```python
from build123d import *

# Parameters (mm, degrees)
F2_R     = 4.2169292551
F3_DEPTH = 41.402
F4_R     = 3.4205639175
F5_DEPTH = 25.4
F6_W     = 9.9848257378
F6_H     = 8.4082745016
F7_DEPTH = 41.402
F8_W     = 6.5733380616
F8_H     = 5.3974576294
F9_DEPTH = 25.4


# Not quite as in the source:
# - the program builds the solid bodies; features that only make, move or delete a surface that nothing else refers to are left out


with BuildPart() as f3:
    # F2 (on Right) → F3 (new body)
    with BuildSketch(Plane.YZ):
        with Locations((0, -23.187154904)):
            Circle(F2_R)
    extrude(amount=F3_DEPTH)

    # F4 (on face) → F5 (cut)
    with BuildSketch(Plane.YZ.offset(41.402)):
        with Locations((0, -23.187154904)):
            Circle(F4_R)
    extrude(amount=-F5_DEPTH, mode=Mode.SUBTRACT)

    # F6 (on Right) → F7 (join)
    with BuildSketch(Plane.YZ):
        with Locations((0, -23.9110346884)):
            Rectangle(F6_W, F6_H)
    extrude(amount=-F7_DEPTH)

    # F8 (on face) → F9 (cut)
    with BuildSketch(Plane(origin=(-41.402, 0, 0), x_dir=(0, -1, 0), z_dir=(-1, 0, 0))):
        with Locations((0, -23.9110346884)):
            Rectangle(F8_W, F8_H)
    extrude(amount=-F9_DEPTH, mode=Mode.SUBTRACT)


solid = f3.part
```
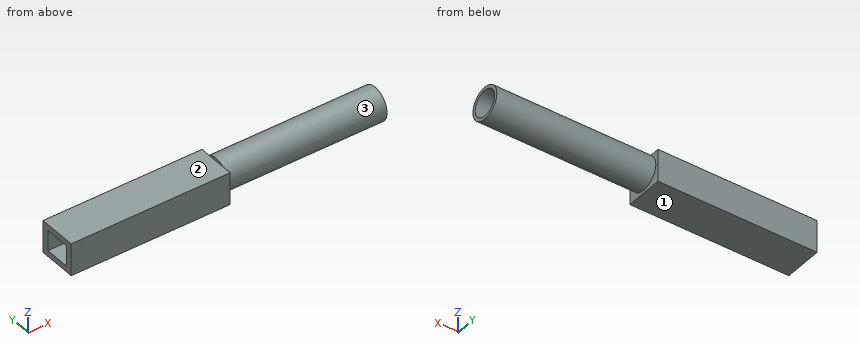
The listing builds one solid part. Answer for the finished solid, in the listing's coordinates (mm). Face numbers are marked on the shaded views. A direction names the side the tool comes from. Round coordinates to 2 decimals unless told otherwise and drop trailing zeros. Write each loop counter-clockwise with the first axis right and the second up, starting at its lowest first coordinate (ties: lowest second). Pieces come first, ordered by that corner, then holes. Notation, with made-up numbers: (70.5, -15) -> (126.5, -15) arc R13 cw to (126.5, -10) -> close; hole circle Ø6 at (53.5, 2.25). An arc over 180 degrees is marked (long way). Answer as a JSON object with one key per item and string values. Group by question number.
Q1. Section B-B (y = 0) is taken. Write down the section's boundary in (x, z).
Q2. Section C-C (z = -20.5) is taken. Write down the section's boundary in (x, y), plus the area to 3 significant figures.
Q3. Which of the six approach directions +Z, -Z, +X, -X, +Y, -Y give full straight-line access (tool end or side, diameter ignored) to the marked faces 1, 2 and 3?
Q4. Section A-A (x = -30) is taken. Write down the section's boundary in (y, z), plus the area to 3 significant figures.
Q5. Section D-D (x = -12) is taken. Write down the section's boundary in (y, z).
Q6. Each of these flat-tipped pins is pushed along its axis until it touches: pin 1 Ø1.6 at (y, z) = (-0.5, -23) entering from -X; pin 2 Ø3.5 at (x, y) = (-26, 0) entering from +Z; pin 3 Ø1 at (x, y) = (29.5, 1) entering from +Z. Where does it stop, or does it pass through?
Q7. Straight lines are drawn through the part: line 1 along Y through (x, z) = (-19, -21.75); line 2 along Z through (x, y) = (29.5, 0); line 3 along X through (y, z) = (-3.5, -27). For each, find the intervals that lie inside material, in ascending order.
Check values:
{
 "1": {"outline": "(-41.4, -28.12) -> (0, -28.12) -> (0, -27.4) -> (41.4, -27.4) -> (41.4, -26.61) -> (16, -26.61) -> (16, -19.77) -> (41.4, -19.77) -> (41.4, -18.97) -> (0, -18.97) -> (0, -19.71) -> (-41.4, -19.71) -> (-41.4, -21.21) -> (-16, -21.21) -> (-16, -26.61) -> (-41.4, -26.61) -> close"},
 "2": {"outline": "(-41.4, -4.99) -> (0, -4.99) -> (0, -3.25) -> (41.4, -3.25) -> (41.4, -2.12) -> (16, -2.12) -> (16, 2.12) -> (41.4, 2.12) -> (41.4, 3.25) -> (0, 3.25) -> (0, 4.99) -> (-41.4, 4.99) -> close", "area": "575 mm^2"},
 "3": {"face 1": "-Z, +X, -X, +Y, -Y", "face 2": "+Z, -X, +Y, -Y", "face 3": "+X"},
 "4": {"outline": "(-4.99, -28.12) -> (4.99, -28.12) -> (4.99, -19.71) -> (-4.99, -19.71) -> close; hole (-3.29, -26.61) -> (3.29, -26.61) -> (3.29, -21.21) -> (-3.29, -21.21) -> close", "area": "48.5 mm^2"},
 "5": {"outline": "(-4.99, -28.12) -> (4.99, -28.12) -> (4.99, -19.71) -> (-4.99, -19.71) -> close"},
 "6": {"pin 1": "x = -16", "pin 2": "z = -19.71", "pin 3": "z = -19"},
 "7": {"line 1": "-4.99 to -3.29, 3.29 to 4.99", "line 2": "-27.4 to -26.61, -19.77 to -18.97", "line 3": "-41.4 to 0"}
}
